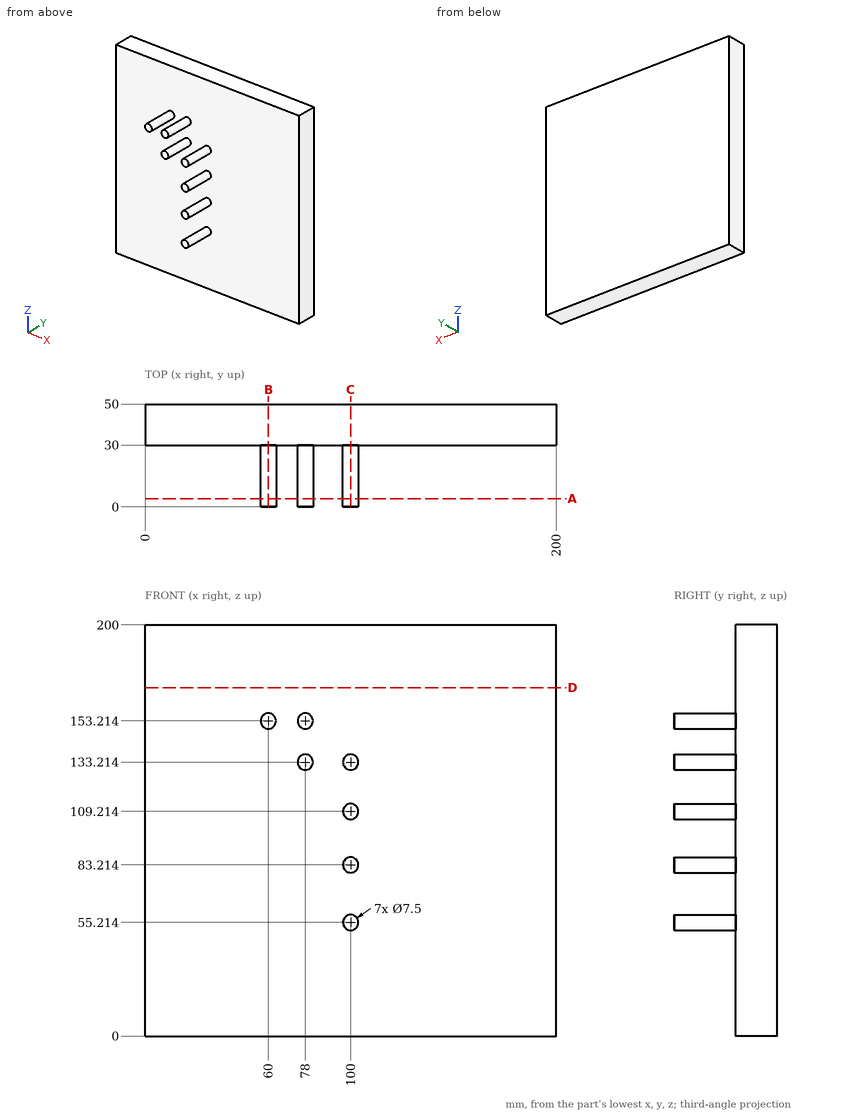
Source: three-view drawing plus pictorial views. Frame: mm from the lowest corner of the part. Round coordinates to 2 decimals unless told otherwise and drop trailing zeros. Loops run counter-clockwise (first coordinate to the right, second up) from the corner with the lowest first, then second, coordinate; pieces in that order, holes last.
1. Contact query for flat-ended pins moving along their axis: pin 1 (10 mm diameter, centred on y = 31.5, z = 142.5, fed in from -X); pin 2 (3 mm diameter, centred on x = 99.5, y = 23.5, fed in from -Z); pin 3 (4 mm diameter, centred on y = 17.5, z = 50, fed in from +X). Output: stop coordinate, or through.
2. Section query D-D on z = 169.5. Output: boundary loops of the cut face in (x, y), and give its area (3 significant figures).
3. Section query C-C on x = 100. Output: boundary loops of the cut face in (y, z) (1 decimal).
4. Section query B-B on x = 60. Output: boundary loops of the cut face in (y, z) (1 decimal), and give its area (4 significant figures).
5. Section query A-A on y = 4. Give the number of separate pieces and of enclosed holes in the cut face, and give its area (3 significant figures).
6. Ray query, L1, parallel to Y at x = 14, z = 144. Return the intervals inside material, ascending.
Answers below:
1. pin 1: stops at x = 0
1. pin 2: stops at z = 51.46
1. pin 3: stops at x = 101.93
2. outline: (0, 30) - (200, 30) - (200, 50) - (0, 50) - close
2. area: 4,000 mm2
3. outline: (0, 51.5) - (30, 51.5) - (30, 0) - (50, 0) - (50, 200) - (30, 200) - (30, 137) - (0, 137) - (0, 129.5) - (30, 129.5) - (30, 113) - (0, 113) - (0, 105.5) - (30, 105.5) - (30, 87) - (0, 87) - (0, 79.5) - (30, 79.5) - (30, 59) - (0, 59) - close
4. outline: (0, 149.5) - (30, 149.5) - (30, 0) - (50, 0) - (50, 200) - (30, 200) - (30, 157) - (0, 157) - close
4. area: 4,225 mm2
5. separate pieces: 7
5. enclosed holes: 0
5. area: 309 mm2
6. L1: y = 30 to 50
